Build history of the part. All positions in model axes, mm. A direction names the side the tool comes from. Coordinates: 2 decimals unless noted, no trailing zeros. Loops run counter-clockwise (first coordinate to the right, second up) from the corner with the lowest first, then second, coordinate; pieces in that order, holes last. Notation, with made-up numbers: (10.25, -33) -> (18.25, -33) arc R9 ccw to (18.25, -29) -> close; hole circle Ø10 at (57.5, 36.5). An arc over 180 degrees is marked (long way). One line per item, written item: value. Start each with the question number.
```python
from build123d import *

# Parameters (mm, degrees)
EXTRUDE_1294_DEPTH   = 1
SKETCH_1344_R        = 1.5
EXTRUDE_1_DEPTH      = 1.5
EXTRUDE_START        = 4
SKETCH_1505_R        = 1.5
EXTRUDE_2_DEPTH      = 4
EXTRUDE_3_DEPTH      = 1.8
EXTRUDE_3_DEPTH_BACK = 1.8
SKETCH_1641_W        = 2
SKETCH_1641_H        = 0.8
CUT_EXTRUDE_START    = -2
CUT_EXTRUDE_1_DEPTH  = 2
SKETCH_6_W           = 1.7
SKETCH_6_H           = 1.7
CUT_EXTRUDE_2_DEPTH  = 2
FILLET_1_R           = 0.3


# Read off the part's stored shape, not the designer's step: the extrude step
with BuildPart() as part:
    # Sketch 213 → Extrude 1294 (new body)
    with BuildSketch(Plane(origin=(0, 0, 0), x_dir=(1, 0, 0), z_dir=(0, 1, 0))):
        with BuildLine():
            Line((-2.5, -2.4), (2.5, -2.4))
            ThreePointArc((2.5, -2.4), (4.9, 0), (2.5, 2.4))
            Line((2.5, 2.4), (-2.5, 2.4))
            ThreePointArc((-2.5, 2.4), (-4.9, 0), (-2.5, -2.4))
        make_face()
    extrude(amount=EXTRUDE_1294_DEPTH)

    # Sketch 1344 → Extrude 1 (add)
    with BuildSketch(Plane(origin=(0, 1, 0), x_dir=(1, 0, 0), z_dir=(0, 1, 0))):
        with Locations(Location((0, 0, 0), (0, 0, 270))):
            Circle(SKETCH_1344_R)
    extrude(amount=EXTRUDE_1_DEPTH)

    # Sketch 1505 → Extrude 2 (add)
    with BuildSketch(Plane.XZ.offset(EXTRUDE_START)):
        with Locations(Location((0, 0, 0), (0, 0, 90))):
            Circle(SKETCH_1505_R)
    extrude(amount=-EXTRUDE_2_DEPTH)

    # Sketch 1641 → Extrude 3 (add, two sides: drawn at the far end of the back side and taken through both)
    with BuildSketch(Plane.XY.offset(-EXTRUDE_3_DEPTH_BACK)):
        with Locations((0, -1.6)):
            Rectangle(SKETCH_1641_W, SKETCH_1641_H)
    extrude(amount=EXTRUDE_3_DEPTH + EXTRUDE_3_DEPTH_BACK)

    # Cut-Extrude 1 outline → Cut-Extrude 1 (cut)
    with BuildSketch(Plane(origin=(1, 0, 0), x_dir=(0, 0, -1), z_dir=(1, 0, 0)).offset(CUT_EXTRUDE_START)):
        with BuildLine():
            ThreePointArc((1.5, -1.2), (1.716666667, -1.35), (1.8, -1.6))
            Line((1.8, -1.6), (1.8, -1.2))
            Line((1.8, -1.2), (1.5, -1.2))
        make_face()
        with BuildLine():
            ThreePointArc((1.8, -1.6), (1.716666667, -1.85), (1.5, -2))
            Line((1.5, -2), (1.8, -2))
            Line((1.8, -2), (1.8, -1.6))
        make_face()
        with BuildLine():
            ThreePointArc((-1.5, -2), (-1.716666667, -1.85), (-1.8, -1.6))
            Line((-1.8, -1.6), (-1.8, -2))
            Line((-1.8, -2), (-1.5, -2))
        make_face()
        with BuildLine():
            ThreePointArc((-1.8, -1.6), (-1.716666667, -1.35), (-1.5, -1.2))
            Line((-1.5, -1.2), (-1.8, -1.2))
            Line((-1.8, -1.2), (-1.8, -1.6))
        make_face()
    extrude(amount=CUT_EXTRUDE_1_DEPTH, mode=Mode.SUBTRACT)

    # Sketch 6 → Cut-Extrude 2 (cut)
    with BuildSketch(Plane.XZ.offset(4)):
        Rectangle(SKETCH_6_W, SKETCH_6_H)
    extrude(amount=-CUT_EXTRUDE_2_DEPTH, mode=Mode.SUBTRACT)

    # Fillet 1
    fillet_1_edges = [part.edges().sort_by_distance(p)[0] for p in [
        (0, 2.5, -1.5),
        (1, -1.2, 1.309016994),
        (1, -2, 1.309016994),
        (-1, -2, 1.309016994),
        (-1, -1.2, 1.309016994),
        (-1, -2, -1.309016994),
        (1, -2, -1.309016994),
        (-1, -1.85, 1.716666667),
        (1, -1.85, 1.716666667),
        (-1, -1.35, -1.716666667),
        (1, -1.35, -1.716666667),
        (1, -1.2, -1.309016994),
        (-1, -1.2, -1.309016994),
    ]]
    fillet(fillet_1_edges, radius=FILLET_1_R)


solid = part.part
```
Item 1: Band-saw the part on B-B, the plane y = 1.5. List the corners of the cut face in (x, z).
Item 2: Probe probe 1 along Y at (x, z) = (-3, 0.15); probe 2 along X at (y, z) = (1.25, 0.4); probe 3 along Y at (x, z) = (0.5, -0.4). List the from-to ranges inside material, lowest first.
Item 3: Band-saw the part on C-C, the plane z = -2. List the corners of the cut face in (x, y), and give its area (3 significant figures).
Item 4: Drop flat-ended pins along their axis: pin 1 Ø1.5 at (y, z) = (-3, 0) entering from +X; pin 2 Ø0.5 at (x, y) = (-0.5, -3) entering from +Z; pin 3 Ø1.4 at (y, z) = (-3, -0.5) entering from -X; pin 4 Ø2.5 at (x, z) = (2, -0.5) entering from -Y. Give the stop position or say it passes through.
Item 5: Two-plate mould, pull along X, no slides. Class faces 1 (the face through (0, 0, 2)), 2 (the face through (-4.9, 0.49, -0.05)), 3 (the face through (0, -3, 0.85)): +X half, -X half, draft (parallel to the pull), parting line (faces both ways), or undercut.
Item 6: Tool access for faces 4 (the face through (-0.85, -3, 0)), 5 (the face through (0, 0.5, 2.4)), 6 (the face through (-1.487, -2.028, -0.195)), 7 (the face through (0.45, 1.59, 1.43)): list every direction of +Z, -Z, +X, -X, +Y, -Y with a clear straight run to the whole face (end or side of a thin tool).
Item 7: Band-saw the part on A-A, the plane z = 0. List the corners of the cut face in (x, y).
Worked out:
1. outline: circle Ø3 at (0, 0)
2. probe 1: y = 0 to 1
2. probe 2: x = -1.45 to 1.45
2. probe 3: y = -2 to 2.5
3. outline: (-3.83, 0) -> (3.83, 0) -> (3.83, 1) -> (-3.83, 1) -> close
3. area: 7.65 mm²
4. pin 1: stops at x = 1.5
4. pin 2: stops at z = 1.48
4. pin 3: stops at x = -1.5
4. pin 4: stops at y = -4
5. face 1: draft
5. face 2: -X half
5. face 3: undercut
6. face 4: -Y
6. face 5: +Z, +X, -X, +Y, -Y
6. face 6: none
6. face 7: +Y
7. outline: (-4.9, 0) -> (-1.5, 0) -> (-1.5, -4) -> (-0.85, -4) -> (-0.85, -2) -> (0.85, -2) -> (0.85, -4) -> (1.5, -4) -> (1.5, 0) -> (4.9, 0) -> (4.9, 1) -> (1.5, 1) -> (1.5, 2.2) arc R0.3 ccw to (1.2, 2.5) -> (-1.2, 2.5) arc R0.3 ccw to (-1.5, 2.2) -> (-1.5, 1) -> (-4.9, 1) -> close
